Part print with two shaded views. Sizes in mm from the minimum x, y, z corner. Coordinates: 2 decimals unless noted, no trailing zeros. Write each loop counter-clockwise with the first axis right and the second up, starting at its lowest first coordinate (ties: lowest second). Pieces come first, ordered by that corner, then holes. Notation, with made-up numbers: (-10.5, 77.5) - (42.5, 77.5) arc R34 cw to (42.5, 114.5) - close; hole circle Ø2 at (44, 5). An arc over 180 degrees is marked (long way). One line per question, with ' | ' between items. Start each with the question number.
1. Band-saw the part on A-A, the plane y = 7.5. Write the cut outline in (x, z).
2. Band-saw the part on B-B, the plane x = 145. Write the cut outline in (y, z) (3 decimals), then the cut area to 4 significant figures.
3. Probe line 1 (Y direction, x = 248, z = 5) (3 decimals); line 2 (Y direction, x = 306, z = 2.75); line 3 (X direction, y = 40.5, z = 3). List the from-to ranges inside material, lowest first.
4. Flat gauge pins, fed straight in: P1, Ø5, axis at y = 8, z = 4.5, coming from the -X side; P2, Ø2, axis at y = 38, z = 7.5, coming from the -X side. Where does each tip first touch, or does it go through?
5. Band-saw the part on C-C, the plane z = 4. Write the cut outline in (x, y) (3 decimals).
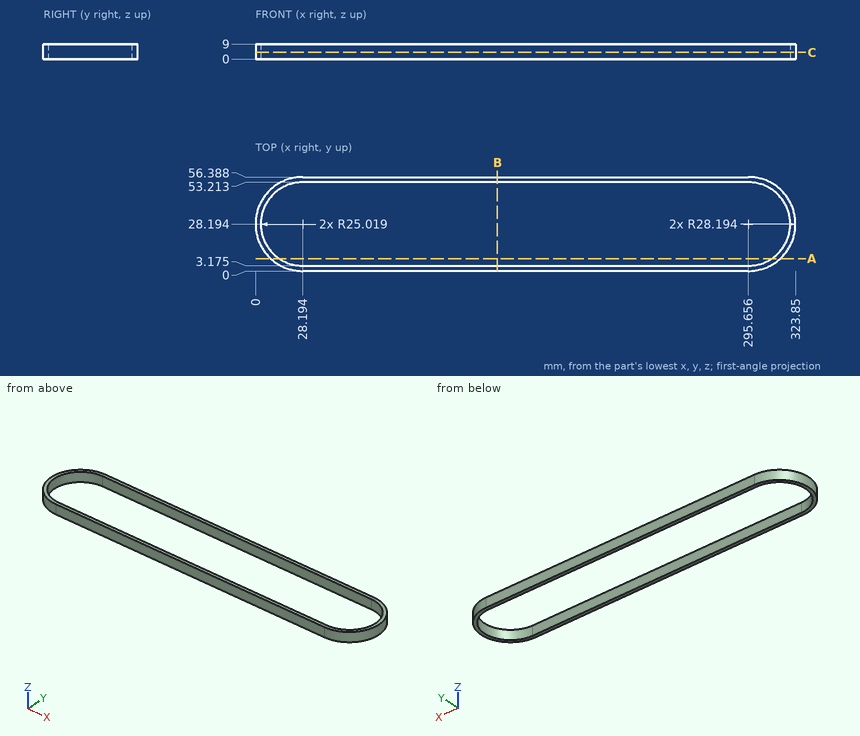
Filled in:
1) outline: (9.05, 0) - (14.13, 0) - (14.13, 9) - (9.05, 9) - close; (309.72, 0) - (314.8, 0) - (314.8, 9) - (309.72, 9) - close
2) outline: (0, 0) - (3.175, 0) - (3.175, 9) - (0, 9) - close; (53.213, 0) - (56.388, 0) - (56.388, 9) - (53.213, 9) - close | area: 57.15 mm²
3) line 1: y = 0 to 3.175, 53.213 to 56.388 | line 2: y = 1.97 to 5.41, 50.97 to 54.42 | line 3: x = 2.83 to 6.41, 317.44 to 321.02
4) P1: stops at x = 6.24 | P2: stops at x = 1.41
5) outline: (28.194, 0) - (295.656, 0) arc R28.194 ccw to (295.656, 56.388) - (28.194, 56.388) arc R28.194 ccw to start; hole (28.194, 3.175) - (295.656, 3.175) arc R25.019 ccw to (295.656, 53.213) - (28.194, 53.213) arc R25.019 ccw to start
